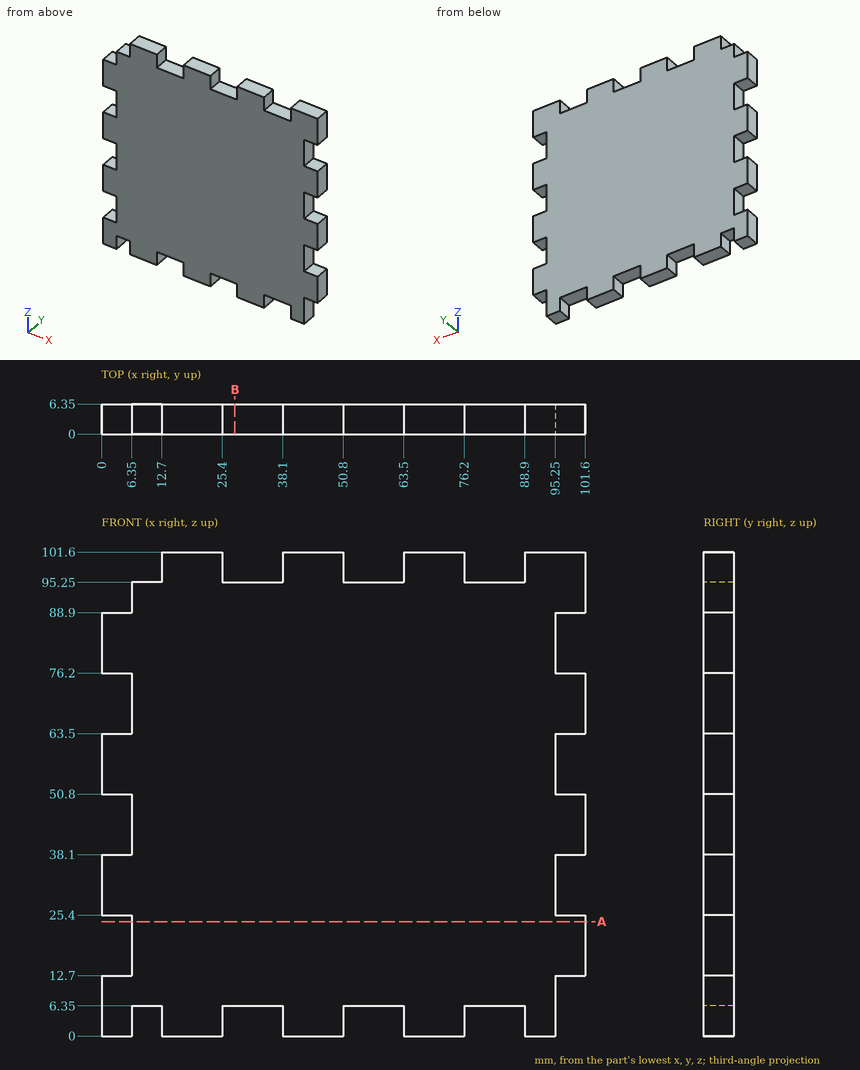
Here's the drawing with two shaded views (mm, measured from the low corner). I have some questions. Coordinates: 2 decimals unless noted, no trailing zeros. Loops run counter-clockwise (first coordinate to the right, second up) from the corner with the lowest first, then second, coordinate; pieces in that order, holes last. Notation, with made-up numbers: (10, 26) -> (38, 26) arc R11 ccw to (38, 45) -> close; hole circle Ø4 at (-13.75, -27). An arc over 180 degrees is marked (long way). Answer as a JSON object with one key per item and string values.
1) Imagine slicing it at A-A (z = 24). Please give me the cut outline in (x, y), then the cut area to 3 significant figures.
Results:
{"outline": "(6.35, 0) -> (101.6, 0) -> (101.6, 6.35) -> (6.35, 6.35) -> close", "area": "605 mm^2"}
2) If I drill on line 1 (X direction, y = 2.5, z = 6); line 2 (Z direction, x = 5, y = 3.75); line 3 (Z direction, x = 35, y = 2.5), over which ranges is the centre line in solid material (lowest first)?
Results:
{"line 1": "x = 0 to 6.35, 12.7 to 25.4, 38.1 to 50.8, 63.5 to 76.2, 88.9 to 95.25", "line 2": "z = 0 to 12.7, 25.4 to 38.1, 50.8 to 63.5, 76.2 to 88.9", "line 3": "z = 6.35 to 95.25"}
3) For P1, Ø1.9, axis at x = 80, y = 2, coming from the +Z side; P2, Ø3, axis at x = 3, y = 3, coming from the +Z side; P3, Ø1.9, axis at y = 2.5, z = 1.5, coming from the +X side, each with a flat end and sliding along its axis, tell me the tip position at first contact or that it passes through.
Results:
{"P1": "stops at z = 95.25", "P2": "stops at z = 88.9", "P3": "stops at x = 95.25"}
4) Imagine slicing it at B-B (x = 28). Please give me the cut outline in (y, z).
Results:
{"outline": "(0, 6.35) -> (6.35, 6.35) -> (6.35, 95.25) -> (0, 95.25) -> close"}
